CAD build for the part. Positions are in the model's coordinates, mm. A direction names the side the tool comes from. Give positions to 0.01 mm unless a question says otherwise; leave off trailing zeros. Loops run counter-clockwise (first coordinate to the right, second up) from the corner with the lowest first, then second, coordinate; pieces in that order, holes last. Notation, with made-up numbers: (43, 22) -> (87, 22) arc R15 cw to (87, 33) -> close; hole circle Ø2 at (60.25, 0). An arc over 180 degrees is marked (long way). Use one line per item in the form item = value.
```python
from build123d import *

# Parameters (mm, degrees)
BOSS_EXTRUDE1_DEPTH = 6
SKETCH2_R           = 2
CUT_EXTRUDE1_DEPTH  = 71.989922019


with BuildPart() as part:
    # Sketch1 → Boss-Extrude1 (new body)
    with BuildSketch(Plane(origin=(0, 0, 0), x_dir=(1, 0, 0), z_dir=(0, 1, 0))):
        Polygon((4.371579812, 18.793220339), (4.371579812, 58.793220339), (-14.628420188, 58.793220339), (-14.628420188, -69.206779661), (4.371579812, -69.206779661), (4.371579812, -29.206779661), (10.371579812, -29.206779661), (10.371579812, 18.793220339), align=None)
    extrude(amount=BOSS_EXTRUDE1_DEPTH)

    # Sketch2 → Cut-Extrude1 (cut, through all)
    with BuildSketch(Plane(origin=(0, 6, 0), x_dir=(1, 0, 0), z_dir=(0, 1, 0))):
        with Locations(Location((-7.128420188, -54.206779661, 0), (0, 0, 270))):
            Circle(SKETCH2_R)
        with Locations(Location((-7.128420188, 43.793220339, 0), (0, 0, 270))):
            Circle(SKETCH2_R)
    extrude(amount=-CUT_EXTRUDE1_DEPTH, mode=Mode.SUBTRACT)


solid = part.part
```
1. Cut at C-C, the plane x = 6. Write the cut outline in (y, z), then the cut area to 3 significant figures.
Result sheet:
outline = (0, -18.79) -> (6, -18.79) -> (6, 29.21) -> (0, 29.21) -> close
area = 288 mm^2
2. Mould opens along Z. For faces 1 (the cylindrical face through (-7.894, 3.042, 56.054)), 2 (the flat face through (7, 3, -18.793)), 3 (the cylindrical face through (-7.894, 3.042, -41.946)), 4 (the flat face through (-5, 6, 4)) say: pulls with the +Z half, pulls with the -Z half, needs draft (parallel to the pull), parting line crosses it, or undercut.
Result sheet:
face_1 = undercut
face_2 = pulls with the -Z half
face_3 = undercut
face_4 = needs draft
3. Drill centre lines: line 1 (Z direction, x = -7, y = 2.65); line 2 (X direction, y = 4.2, z = 45); line 3 (Z direction, x = 8, y = 2.8). Where is each one in solid material? Low to high.
Result sheet:
line_1 = -58.79 to -45.79, -41.8 to 52.21, 56.2 to 69.21
line_2 = -14.63 to 4.37
line_3 = -18.79 to 29.21
4. Cut at B-B, the plane z = 46.5. Write the cut outline in (x, y), then the cut area to 3 significant figures.
Result sheet:
outline = (-14.63, 0) -> (4.37, 0) -> (4.37, 6) -> (-14.63, 6) -> close
area = 114 mm^2
5. Cut at A-A, the plane y = 2.4. Write the cut outline in (x, z).
Result sheet:
outline = (-14.63, -58.79) -> (4.37, -58.79) -> (4.37, -18.79) -> (10.37, -18.79) -> (10.37, 29.21) -> (4.37, 29.21) -> (4.37, 69.21) -> (-14.63, 69.21) -> close; hole circle Ø4 at (-7.13, -43.79); hole circle Ø4 at (-7.13, 54.21)
6. Tool access for faces 5 (the flat face through (-5, 3, -58.793)), 6 (the flat face through (4.372, 3, 49)), 7 (the flat face through (4.372, 3, -39)): list every direction of +Z, -Z, +X, -X, +Y, -Y with a clear straight run to the whole face (end or side of a thin tool).
Result sheet:
face_5 = -Z, +X, -X, +Y, -Y
face_6 = +Z, +X, +Y, -Y
face_7 = -Z, +X, +Y, -Y
7. Drop flat-ended pins along their axis: P1, Ø3, axis at x = 7, y = 3.5, coming from the -Z side; P2, Ø3, axis at x = 8, y = 2, coming from the +Z side. Give the stop position or say it passes through.
Result sheet:
P1 = -18.79
P2 = 29.21
